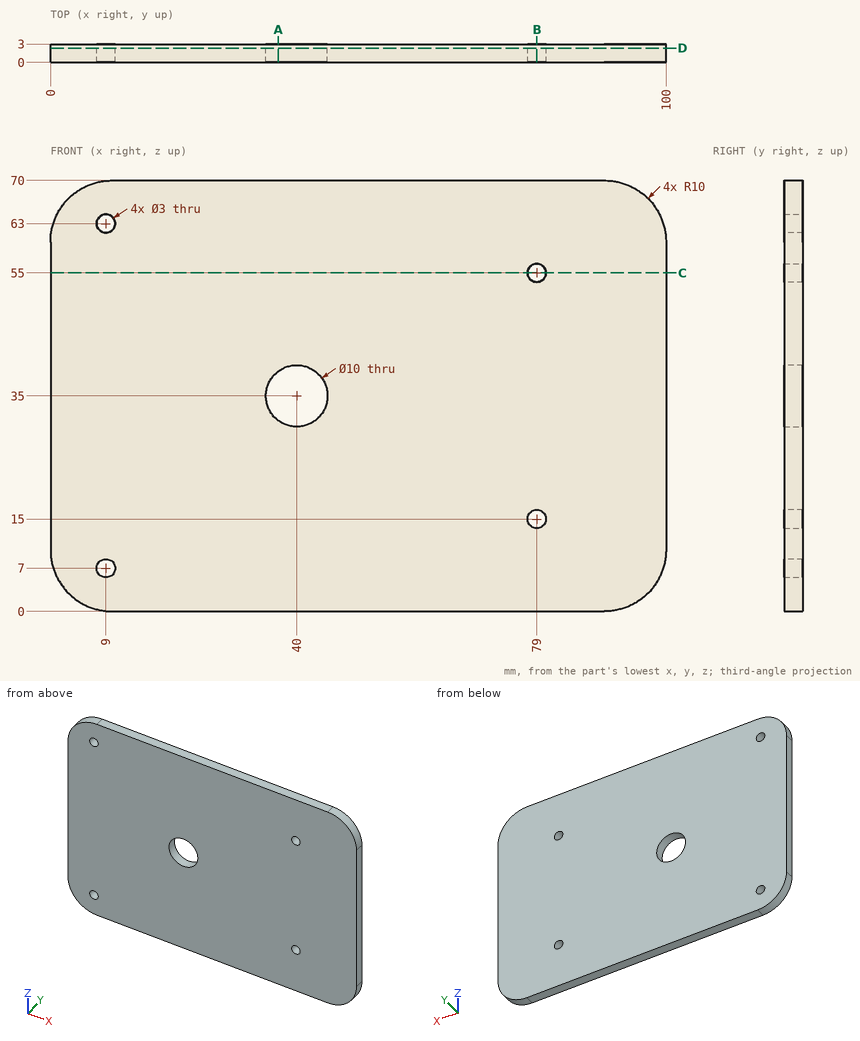
The figure shows three views and two pictorial views of one solid part (mm, origin at its lowest corner). Answer the questions. Coordinates: 2 decimals unless noted, no trailing zeros. Loops run counter-clockwise (first coordinate to the right, second up) from the corner with the lowest first, then second, coordinate; pieces in that order, holes last. Notation, with made-up numbers: (82, 79.5) - (114, 79.5) arc R15 cw to (114, 95.5) - close; hole circle Ø8 at (36, 14.25). An arc over 180 degrees is marked (long way). Write item = value, one per line.
1) Section C-C (z = 55) is taken. Determine the outline of the cut face in (x, y), plus the area to 3 significant figures.
Responses:
outline = (0, 0) - (77.5, 0) - (77.5, 3) - (0, 3) - close; (80.5, 0) - (100, 0) - (100, 3) - (80.5, 3) - close
area = 291 mm^2
2) Section D-D (y = 2.35) is taken. Determine the outline of the cut face in (x, z), plus the area to 3 significant figures.
Responses:
outline = (0, 10) arc R10 ccw to (10, 0) - (90, 0) arc R10 ccw to (100, 10) - (100, 60) arc R10 ccw to (90, 70) - (10, 70) arc R10 ccw to (0, 60) - close; hole circle Ø3 at (9, 7); hole circle Ø3 at (9, 63); hole circle Ø10 at (40, 35); hole circle Ø3 at (79, 15); hole circle Ø3 at (79, 55)
area = 6,810 mm^2
3) Section B-B (x = 79) is taken. Determine the outline of the cut face in (y, z).
Responses:
outline = (0, 0) - (3, 0) - (3, 13.5) - (0, 13.5) - close; (0, 16.5) - (3, 16.5) - (3, 53.5) - (0, 53.5) - close; (0, 56.5) - (3, 56.5) - (3, 70) - (0, 70) - close
4) Find the intervals of material crossed by line 1 along Z through (x, y) = (79, 1.65); line 2 along X through (y, z) = (1.55, 35); line 3 along X through (y, z) = (2.35, 64), in increasing order.
Responses:
line_1 = 0 to 13.5, 16.5 to 53.5, 56.5 to 70
line_2 = 0 to 35, 45 to 100
line_3 = 0.83 to 7.88, 10.12 to 99.17
5) This flat-tipped pin is pushed along its axis until it touches: P1, Ø1.8, axis at x = 9, z = 7, coming from the -Y side. Where does it stop, or does it pass through?
Responses:
P1 = through
6) Section A-A (x = 37) is taken. Determine the outline of the cut face in (y, z), plus the area to 3 significant figures.
Responses:
outline = (0, 0) - (3, 0) - (3, 31) - (0, 31) - close; (0, 39) - (3, 39) - (3, 70) - (0, 70) - close
area = 186 mm^2
